```python
from build123d import *

# Parameters (mm, degrees)
SKETCH_1_R                = 6
EXTRUDE_1_DEPTH           = 50
SKETCH_2_W                = 25
SKETCH_2_H                = 6
EXTRUDE_2_DEPTH           = 50
SKETCH_5_R                = 3
CUT_EXTRUDE_1_DEPTH       = 50
HOLE_WIZARD_1_D           = 6
HOLE_WIZARD_1_CSINK_D     = 12
HOLE_WIZARD_1_CSINK_ANGLE = 90
CUT_EXTRUDE_2_DEPTH       = 12.5
PATTERN_LINEAR_2_COUNT    = 2
PATTERN_LINEAR_2_PITCH    = 25
CHAMFER_1_SIZE            = 2.5


with BuildPart() as part:
    # 草图1 → 凸台-拉伸1 (new body)
    with BuildSketch(Plane.XY):
        with Locations((-36.999696345, 47.332553752)):
            Circle(SKETCH_1_R)
    extrude(amount=EXTRUDE_1_DEPTH)

    # 草图2 → 凸台-拉伸2 (add)
    with BuildSketch(Plane.XY.offset(50)):
        with Locations((-24.499696345, 44.332553752)):
            Rectangle(SKETCH_2_W, SKETCH_2_H)
    extrude(amount=-EXTRUDE_2_DEPTH)

    # 草图5 → 切除-拉伸1 (cut)
    with BuildSketch(Plane.XY.offset(50)):
        with Locations((-36.999696345, 47.332553752)):
            Circle(SKETCH_5_R)
    extrude(amount=-CUT_EXTRUDE_1_DEPTH, mode=Mode.SUBTRACT)

    # 打孔尺寸(%根据)内六角花形半沉头螺钉的类型1 (through all)
    with Locations(Plane(origin=(0, 47.332553752, 0), x_dir=(1, 0, 0), z_dir=(0, 1, 0))):
        with Locations((-21.999696345, -40), (-21.999696345, -10)):
            CounterSinkHole(HOLE_WIZARD_1_D / 2, HOLE_WIZARD_1_CSINK_D / 2, counter_sink_angle=HOLE_WIZARD_1_CSINK_ANGLE)

    # 草图9 → 切除-拉伸2 (cut)
    with BuildSketch(Plane.XY.offset(50)):
        Polygon((-30.999696345, 47.332553752), (-30.999696345, 35.818106439), (-46.000108994, 35.818106439), (-46.000108994, 53.909109131), (-30.999696345, 53.909109131), align=None)
    cut_extrude_2 = extrude(amount=-CUT_EXTRUDE_2_DEPTH, mode=Mode.SUBTRACT)

    # 阵列(线性)2: 切除-拉伸2 ×2
    with Locations(*[(0, 0, -i * PATTERN_LINEAR_2_PITCH) for i in range(1, PATTERN_LINEAR_2_COUNT)]):
        add(cut_extrude_2, mode=Mode.SUBTRACT)

    # 倒角1
    chamfer_1_edges = [part.edges().sort_by_distance(p)[0] for p in [
        (-11.999696345, 47.332553752, 25),
    ]]
    chamfer(chamfer_1_edges, length=CHAMFER_1_SIZE)


solid = part.part
```
The listing builds one solid part. Answer for the finished solid, in the listing's coordinates (mm). A direction names the side the tool comes from. Give positions to 0.01 mm unless a question says otherwise; leave off trailing zeros. Loops run counter-clockwise (first coordinate to the right, second up) from the corner with the lowest first, then second, coordinate; pieces in that order, holes last. Notation, with made-up numbers: (-14.5, 40.5) - (27.5, 40.5) arc R20 ccw to (27.5, 51.5) - close; hole circle Ø3 at (-4, -37.5). An arc over 180 degrees is marked (long way). Return JSON: item names as keys, results as strings. Group by question number.
1. Find section B-B (z = 40). Write down the section's boundary in (x, y).
2. Given pin 1 Ø9.5 at (x, z) = (-22, 40) entering from +Y; pin 2 Ø6 at (x, y) = (-35.5, 50) entering from +Z; pin 3 Ø5 at (x, z) = (-22, 10) entering from +Y; pin 4 Ø3 at (y, z) = (43.5, 46) entering from -X, each flat-ended and moving along its own axis, determine where each tip first touches the part or whether it passes through.
3. Which of the six approach directions +Z, -Z, +X, -X, +Y, -Y give full straight-line access (tool end or side, diameter ignored) to faces 4 (the flat face through (-22, 44, 50)), 5 (the flat face through (-23, 47.333, 25)), 6 (the flat face through (-31, 44, 44)), 7 (the flat face through (-34, 46, 12.5))?
4. Determine the mould class of faces 1 (the cylindrical face through (-34.138, 48.234, 6.337)), 2 (the flat face through (-34, 46, 37.5)), 3 (the conical face through (-25, 44.478, 39.055)) for opening direction Z: pulls with the +Z half, pulls with the -Z half, needs draft (parallel to the pull), parting line crosses it, or undercut.
5. Find section C-C (y = 52.25). Write down the section's boundary in (x, z).
6. Find section D-D (z = 26). Write down the section's boundary in (x, y), then the cut area to 3 significant figures.
7. Straight lines are drawn through the part: line 1 (Z direction, x = -42, y = 49.5); line 2 (Z direction, x = -20, y = 45.75); line 3 (X direction, y = 42.25, z = 40). For each, find the intervals that lie inside material, in ascending order. Write a range as [from, to].
8. Find section A-A (z = 10). Write down the section's boundary in (x, y).
Verdict:
{
 "1": {"outline": "(-31, 41.33) - (-25, 41.33) - (-25, 44.33) - (-28, 47.33) - (-31, 47.33) - close; (-19, 41.33) - (-12, 41.33) - (-12, 44.83) - (-14.5, 47.33) - (-16, 47.33) - (-19, 44.33) - close"},
 "2": {"pin 1": "stops at y = 46.08", "pin 2": "stops at z = 37.5", "pin 3": "passes through", "pin 4": "stops at x = -31"},
 "3": {"face 4": "+Z, +X, -X, +Y, -Y", "face 5": "+Z, -Z, +X, +Y", "face 6": "+Z, -X, +Y, -Y", "face 7": "-X, +Y, -Y"},
 "4": {"face 1": "needs draft", "face 2": "pulls with the +Z half", "face 3": "undercut"},
 "5": {"outline": "(-40.44, 0) - (-33.56, 0) - (-33.56, 12.5) - (-40.44, 12.5) - close; (-40.44, 25) - (-33.56, 25) - (-33.56, 37.5) - (-40.44, 37.5) - close"},
 "6": {"outline": "(-37, 41.33) - (-12, 41.33) - (-12, 44.83) - (-14.5, 47.33) - (-31, 47.33) arc R6 ccw (long way) to start; hole circle Ø6 at (-37, 47.33)", "area": "203 mm^2"},
 "7": {"line 1": "z = [0, 12.5], [25, 37.5]", "line 2": "z = [0, 6.06], [13.94, 36.06], [43.94, 50]", "line 3": "x = [-31, -25], [-19, -12]"},
 "8": {"outline": "(-37, 41.33) - (-25, 41.33) - (-25, 44.33) - (-28, 47.33) - (-31, 47.33) arc R6 ccw (long way) to start; (-19, 41.33) - (-12, 41.33) - (-12, 44.83) - (-14.5, 47.33) - (-16, 47.33) - (-19, 44.33) - close; hole circle Ø6 at (-37, 47.33)"}
}
